```python
from build123d import *

# Parameters (mm, degrees)
SKETCH1_W            = 25
SKETCH1_H            = 7.5
BOSS_EXTRUDE1_DEPTH  = 3
CUT_EXTRUDE2_DEPTH   = 4
BOSS_EXTRUDE2_DEPTH  = 3
FILLET8_R            = 2.5
FILLET4_R            = 3.5
M3_CLEARANCE_HOLE1_D = 3.6
FILLET6_R            = 1
FILLET7_R            = 0.25


with BuildPart() as part:
    # Sketch1 → Boss-Extrude1 (new body)
    with BuildSketch(Plane(origin=(0, 0, 0), x_dir=(1, 0, 0), z_dir=(0, 1, 0))):
        Rectangle(SKETCH1_W, SKETCH1_H)
    extrude(amount=BOSS_EXTRUDE1_DEPTH)

    # Sketch1<3> → Cut-Extrude2 (cut, through all)
    with BuildSketch(Plane(origin=(0, 0, 0), x_dir=(1, 0, 0), z_dir=(0, 1, 0))):
        with BuildLine():
            Line((2.456770065, -1.119946806), (1.091049314, -1.10887844))
            Line((1.091049314, -1.10887844), (1.079980948, -2.47459919))
            ThreePointArc((1.079980948, -2.47459919), (-0.021881199, -2.699911334), (-1.119946806, -2.456770065))
            Line((-1.119946806, -2.456770065), (-1.10887844, -1.091049314))
            Line((-1.10887844, -1.091049314), (-2.47459919, -1.079980948))
            ThreePointArc((-2.47459919, -1.079980948), (-2.699911334, 0.021881199), (-2.456770065, 1.119946806))
            Line((-2.456770065, 1.119946806), (-1.091049314, 1.10887844))
            Line((-1.091049314, 1.10887844), (-1.079980948, 2.47459919))
            ThreePointArc((-1.079980948, 2.47459919), (0.021881199, 2.699911334), (1.119946806, 2.456770065))
            Line((1.119946806, 2.456770065), (1.10887844, 1.091049314))
            Line((1.10887844, 1.091049314), (2.47459919, 1.079980948))
            ThreePointArc((2.47459919, 1.079980948), (2.699911334, -0.021881199), (2.456770065, -1.119946806))
        make_face()
        with BuildLine():
            ThreePointArc((-0.818311322, -2.256184075), (-0.019449955, -2.399921186), (0.781636135, -2.269150712))
            Line((0.781636135, -2.269150712), (0.79349041, -0.806457047))
            Line((0.79349041, -0.806457047), (2.256184075, -0.818311322))
            ThreePointArc((2.256184075, -0.818311322), (2.399921186, -0.019449955), (2.269150712, 0.781636135))
            Line((2.269150712, 0.781636135), (0.806457047, 0.79349041))
            Line((0.806457047, 0.79349041), (0.818311322, 2.256184075))
            ThreePointArc((0.818311322, 2.256184075), (0.019449955, 2.399921186), (-0.781636135, 2.269150712))
            Line((-0.781636135, 2.269150712), (-0.79349041, 0.806457047))
            Line((-0.79349041, 0.806457047), (-2.256184075, 0.818311322))
            ThreePointArc((-2.256184075, 0.818311322), (-2.399921186, 0.019449955), (-2.269150712, -0.781636135))
            Line((-2.269150712, -0.781636135), (-0.806457047, -0.79349041))
            Line((-0.806457047, -0.79349041), (-0.818311322, -2.256184075))
        make_face(mode=Mode.SUBTRACT)
        with BuildLine():
            Line((-0.818311322, -2.256184075), (-0.806457047, -0.79349041))
            Line((-0.806457047, -0.79349041), (-2.269150712, -0.781636135))
            ThreePointArc((-2.269150712, -0.781636135), (-2.399921186, 0.019449955), (-2.256184075, 0.818311322))
            Line((-2.256184075, 0.818311322), (-0.79349041, 0.806457047))
            Line((-0.79349041, 0.806457047), (-0.781636135, 2.269150712))
            ThreePointArc((-0.781636135, 2.269150712), (0.019449955, 2.399921186), (0.818311322, 2.256184075))
            Line((0.818311322, 2.256184075), (0.806457047, 0.79349041))
            Line((0.806457047, 0.79349041), (2.269150712, 0.781636135))
            ThreePointArc((2.269150712, 0.781636135), (2.399921186, -0.019449955), (2.256184075, -0.818311322))
            Line((2.256184075, -0.818311322), (0.79349041, -0.806457047))
            Line((0.79349041, -0.806457047), (0.781636135, -2.269150712))
            ThreePointArc((0.781636135, -2.269150712), (-0.019449955, -2.399921186), (-0.818311322, -2.256184075))
        make_face()
    extrude(amount=CUT_EXTRUDE2_DEPTH, mode=Mode.SUBTRACT)

    # Sketch4 → Boss-Extrude2 (add)
    with BuildSketch(Plane(origin=(0, 0, 0), x_dir=(1, 0, 0), z_dir=(0, 1, 0))):
        with BuildLine():
            Line((-4.683748499, 3.75), (4.683748499, 3.75))
            ThreePointArc((4.683748499, 3.75), (0, 6), (-4.683748499, 3.75))
        make_face()
        with BuildLine():
            ThreePointArc((-4.683748499, -3.75), (0, -6), (4.683748499, -3.75))
            Line((4.683748499, -3.75), (-4.683748499, -3.75))
        make_face()
    extrude(amount=BOSS_EXTRUDE2_DEPTH)

    # Fillet8
    fillet8_edges = [part.edges().sort_by_distance(p)[0] for p in [
        (-4.683748499, 1.5, -3.75),
        (4.683748499, 1.5, -3.75),
        (4.683748499, 1.5, 3.75),
        (-4.683748499, 1.5, 3.75),
    ]]
    fillet(fillet8_edges, radius=FILLET8_R)

    # Fillet4
    fillet4_edges = [part.edges().sort_by_distance(p)[0] for p in [
        (-12.5, 1.5, 3.75),
        (-12.5, 1.5, -3.75),
        (12.5, 1.5, 3.75),
        (12.5, 1.5, -3.75),
    ]]
    fillet(fillet4_edges, radius=FILLET4_R)

    # M3 Clearance Hole1 (through all)
    with Locations(Plane.XZ):
        with Locations((-7.5, 0), (7.5, 0)):
            Hole(M3_CLEARANCE_HOLE1_D / 2)

    # Fillet6
    fillet6_edges = [part.edges().sort_by_distance(p)[0] for p in [
        (0, 3, 6),
        (0, 0, 6),
        (7.380429655, 0, 3.75),
        (7.380429655, 3, 3.75),
        (0, 3, -6),
        (0, 0, -6),
        (7.380429655, 0, -3.75),
        (7.380429655, 3, -3.75),
        (-4.851350717, 0, 3.921310644),
        (-4.851350717, 3, 3.921310644),
        (4.851350717, 0, 3.921310644),
        (4.851350717, 3, 3.921310644),
        (4.851350717, 0, -3.921310644),
        (4.851350717, 3, -3.921310644),
        (-4.851350717, 0, -3.921310644),
        (-4.851350717, 3, -3.921310644),
        (-7.380429655, 0, 3.75),
        (-12.5, 0, 0),
        (-7.380429655, 0, -3.75),
        (12.5, 0, 0),
        (-11.474873734, 0, -2.724873734),
        (-11.474873734, 0, 2.724873734),
        (11.474873734, 0, 2.724873734),
        (11.474873734, 0, -2.724873734),
        (12.5, 3, 0),
        (-7.380429655, 3, 3.75),
        (-7.380429655, 3, -3.75),
        (-12.5, 3, 0),
        (-11.474873734, 3, -2.724873734),
        (-11.474873734, 3, 2.724873734),
        (11.474873734, 3, 2.724873734),
        (11.474873734, 3, -2.724873734),
    ]]
    fillet(fillet6_edges, radius=FILLET6_R)

    # Fillet7
    fillet7_edges = [part.edges().sort_by_distance(p)[0] for p in [
        (1.091049314, 1.5, 1.10887844),
        (1.10887844, 1.5, -1.091049314),
        (-1.091049314, 1.5, -1.10887844),
        (-1.10887844, 1.5, 1.091049314),
    ]]
    fillet(fillet7_edges, radius=FILLET7_R)


solid = part.part
```
Geometry check sheet. Reference: the model listing, model coordinates, mm. A direction names the side the tool comes from. Round coordinates to 2 decimals unless told otherwise and drop trailing zeros. Loops run counter-clockwise (first coordinate to the right, second up) from the corner with the lowest first, then second, coordinate; pieces in that order, holes last. Notation, with made-up numbers: (-33.5, -39.5) - (-24.5, -39.5) arc R21 cw to (-24.5, -16.5) - close; hole circle Ø1 at (46.5, 67). An arc over 180 degrees is marked (long way). Write each question's results on one line, items separated by ' | '. Start each with the question number.
Q1. Cross-section at A-A on z = 0. Enter the section's corners in (x, y).
Q2. Gauge pin test, flat ends, axial feed: P1, Ø1.1, axis at x = 7.5, y = 1.5, coming from the -Z side; P2, Ø1.5, axis at x = 4.5, y = 1.5, coming from the +Z side; P3, Ø0.5, axis at x = -7, y = 1.5, coming from the +Z side; P4, Ø2, axis at x = -7.5, z = 0, coming from the +Y side. Record the tip position at first contact, or that the pin passes through.
Q3. Cross-section at D-D on x = -8.5. Enter the section's corners in (y, z).
Q4. Access from +Z, -Z, +X, -X, +Y, -Y to the whole of each face (thin tool, end or side, straight path). Record for faces 1 (the cylindrical face through (7.358, 0.285, -3.449)), 2 (the cylindrical face through (-7.403, 0.285, -3.449)), 3 (the cylindrical face through (7.403, 0.285, 3.449)), 4 (the cylindrical face through (7.403, 2.715, 3.449)).
Q5. Thickness scan on line 1 (X direction, y = 2.6, z = -1); line 2 (Z direction, x = -7.5, y = 1.45); line 3 (X direction, y = 1.1, z = 1.5). Record the ranges inside material, lowest first. Write a range as [from, to].
Q6. Cross-section at B-B on x = 7.5. Enter the section's corners in (y, z).
Q7. Cross-section at C-C on y = 1.25. State how many separate pieces and enclosed holes the cut face has, and give its area (3 significant figures).
Answers below:
1) outline: (-12.5, 1) arc R1 ccw to (-11.5, 0) - (-9.3, 0) - (-9.3, 3) - (-11.5, 3) arc R1 ccw to (-12.5, 2) - close; (-5.7, 0) - (-2.7, 0) - (-2.7, 3) - (-5.7, 3) - close; (2.7, 0) - (5.7, 0) - (5.7, 3) - (2.7, 3) - close; (9.3, 0) - (11.5, 0) arc R1 ccw to (12.5, 1) - (12.5, 2) arc R1 ccw to (11.5, 3) - (9.3, 3) - close
2) P1: stops at z = -3.75 | P2: stops at z = 4.68 | P3: stops at z = 3.75 | P4: passes through
3) outline: (0, -2.75) arc R1 ccw to (1, -3.75) - (2, -3.75) arc R1 ccw to (3, -2.75) - (3, -1.5) - (0, -1.5) - close; (0, 1.5) - (3, 1.5) - (3, 2.75) arc R1 ccw to (2, 3.75) - (1, 3.75) arc R1 ccw to (0, 2.75) - close
4) face 1: -Z, +X, -Y | face 2: -Z, -X, -Y | face 3: +Z, +X, -Y | face 4: +Z, +X, +Y
5) line 1: x = [-12.21, -9], [-6, -2.51], [2.51, 6], [9, 12.21] | line 2: z = [-3.75, -1.8], [1.8, 3.75] | line 3: x = [-12.27, -8.49], [-6.51, -1.11], [1.09, 6.51], [8.49, 12.27]
6) outline: (0, -2.75) arc R1 ccw to (1, -3.75) - (2, -3.75) arc R1 ccw to (3, -2.75) - (3, -1.8) - (0, -1.8) - close; (0, 1.8) - (3, 1.8) - (3, 2.75) arc R1 ccw to (2, 3.75) - (1, 3.75) arc R1 ccw to (0, 2.75) - close
7) separate pieces: 1 | enclosed holes: 3 | area: 168 mm²
